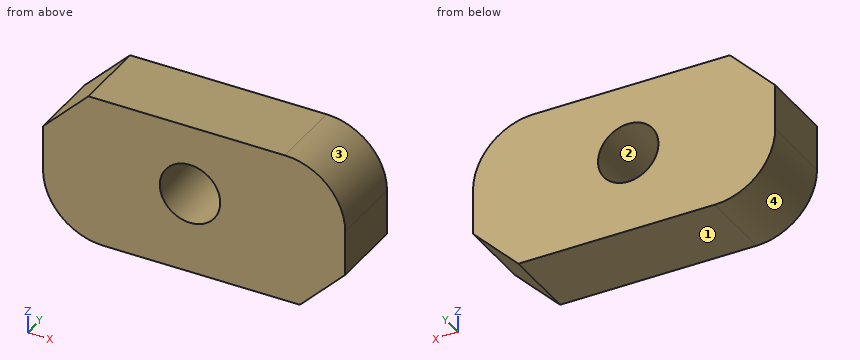
```python
from build123d import *

# Parameters (mm, degrees)
F0_W     = 200
F0_H     = 100
F1_DEPTH = 50
F2_SIZE  = 30
F3_SIZE  = 30
F4_R     = 40
F5_R     = 40
F7_D     = 40


with BuildPart() as f1:
    # F0 (on Front) → F1 (new body)
    with BuildSketch(Plane.XZ):
        with Locations((-100, 50)):
            Rectangle(F0_W, F0_H)
    extrude(amount=F1_DEPTH)

    # F2
    f2_edges = [f1.edges().sort_by_distance(p)[0] for p in [
        (-200, -25, 100),
    ]]
    chamfer(f2_edges, length=F2_SIZE)

    # F3
    f3_edges = [f1.edges().sort_by_distance(p)[0] for p in [
        (0, -25, 0),
    ]]
    chamfer(f3_edges, length=F3_SIZE)

    # F4
    f4_edges = [f1.edges().sort_by_distance(p)[0] for p in [
        (0, -25, 100),
    ]]
    fillet(f4_edges, radius=F4_R)

    # F5
    f5_edges = [f1.edges().sort_by_distance(p)[0] for p in [
        (-200, -25, 0),
    ]]
    fillet(f5_edges, radius=F5_R)

    # F7 (through all)
    with Locations(Plane.XZ.offset(50)):
        with Locations((-102.723882, 53.78725)):
            Hole(F7_D / 2)


solid = f1.part
```
Can you work these out from the model? Positions are in its coordinate system, mm. Face numbers are marked on the shaded views. Coordinates: 2 decimals unless noted, no trailing zeros. Loops run counter-clockwise (first coordinate to the right, second up) from the corner with the lowest first, then second, coordinate; pieces in that order, holes last.
1) For pin 1 (4 mm diameter, centred on x = -173, y = -23.5, fed in from -Z); pin 2 (1.5 mm diameter, centred on y = -19, z = 27.5, fed in from -X); pin 3 (3 mm diameter, centred on x = -84.5, z = 56, fed in from -Y); pin 4 (1.5 mm diameter, centred on y = -38.5, z = 25, fed in from +X), each with a flat end and sliding along its axis, tell me the tip position at first contact or that it passes through.
2) I need wall thicknesses on probe 1 along X at (y, z) = (-41.5, 54.5); probe 2 along X at (y, z) = (-6, 70); probe 3 along Z at (x, y) = (-112, -46). Which ranges of each line are inside material? Lowest first, please.
3) Thinking about a two-plate mould opening in X: for the marked faces 1, 2, 3 and 4, which applies, pulls with the +X half, pulls with the -X half, needs draft (parallel to the pull), parting line crosses it, or undercut?
4) Imagine slicing it at D-D on z = 79. List the corners of the cut face in (x, y) for me, plus the area to 3 significant figures.
5) Imagine slicing it at B-B on z = 57.5. List the corners of the cut face in (x, y) for me, plus the area to 3 significant figures.
6) Imagine slicing it at A-A on x = -107. List the corners of the cut face in (y, z) for me.
7) Imagine slicing it at C-C on y = -32. List the corners of the cut face in (x, z) for me.
Completed:
1. pin 1: stops at z = 1.54
1. pin 2: stops at x = -198.24
1. pin 3: passes through
1. pin 4: stops at x = -4.25
2. probe 1: x = -200 to -122.71, -82.74 to 0
2. probe 2: x = -200 to -114.43, -91.01 to -1.27
2. probe 3: z = 0 to 36.07, 71.51 to 100
3. face 1: needs draft
3. face 2: undercut
3. face 3: pulls with the +X half
3. face 4: pulls with the -X half
4. outline: (-191, -50) - (-4.8, -50) - (-4.8, 0) - (-191, 0) - close
4. area: 9,310 mm2
5. outline: (-200, -50) - (-122.38, -50) - (-122.38, 0) - (-200, 0) - close; (-83.07, -50) - (0, -50) - (0, 0) - (-83.07, 0) - close
5. area: 8,030 mm2
6. outline: (-50, 0) - (0, 0) - (0, 34.25) - (-50, 34.25) - close; (-50, 73.32) - (0, 73.32) - (0, 100) - (-50, 100) - close
7. outline: (-200, 40) arc R40 ccw to (-160, 0) - (-30, 0) - (0, 30) - (0, 60) arc R40 ccw to (-40, 100) - (-170, 100) - (-200, 70) - close; hole circle Ø40 at (-102.72, 53.79)
